```python
from build123d import *

# Parameters (mm, degrees)
BOSS_EXTRUDE1_DEPTH = 3.175
SKETCH3_R           = 1.9685
SKETCH3_R_2         = 1.7018
SKETCH3_R_3         = 1.4605
SKETCH3_R_4         = 1.5875
SKETCH3_R_5         = 1.4732
SKETCH3_R_6         = 1.2065
SKETCH3_W           = 6.5532
SKETCH3_H           = 16.4592
CUT_EXTRUDE1_DEPTH  = 365.434389894


with BuildPart() as part:
    # Sketch1 → Boss-Extrude1 (new body)
    with BuildSketch(Plane(origin=(0, 0, 0), x_dir=(1, 0, 0), z_dir=(0, 1, 0))):
        with BuildLine():
            Line((20.9042, 21.057301381), (20.9042, 9.500301381))
            ThreePointArc((20.9042, 9.500301381), (21.364503799, 7.853774874), (22.611947739, 6.684667206))
            Line((22.611947739, 6.684667206), (32.903843319, 1.321467969))
            add(Edge.make_bspline(
                [(32.903843319, 1.321467969), (33.614873553, 0.950943726), (34.463414094, -1.137550566), (33.907098259, -2.92148302), (32.903843319, -3.444288181)],
                knots=[0, 0, 0, 0, 0.5, 1, 1, 1, 1], degree=3))
            Line((32.903843319, -3.444288181), (22.611947739, -8.807487419))
            ThreePointArc((22.611947739, -8.807487419), (21.364503799, -9.976595087), (20.9042, -11.623121593))
            Line((20.9042, -11.623121593), (20.9042, -27.172610106))
            ThreePointArc((20.9042, -27.172610106), (22.6441, -28.912510106), (24.384, -27.172610106))
            Line((24.384, -27.172610106), (27.051, -27.172610106))
            Line((27.051, -27.172610106), (27.051, -37.859834638))
            ThreePointArc((27.051, -37.859834638), (27.496194931, -39.48118879), (28.706930259, -40.647854028))
            Line((28.706930259, -40.647854028), (80.01, -68.600651316))
            Line((80.01, -68.600651316), (80.01, -252.750651316))
            Line((80.01, -252.750651316), (26.5303, -291.142539353))
            Line((26.5303, -291.142539353), (23.8379, -291.142539353))
            ThreePointArc((23.8379, -291.142539353), (22.1361, -289.440739353), (20.4343, -291.142539353))
            Line((20.4343, -291.142539353), (20.4343, -306.692027866))
            ThreePointArc((20.4343, -306.692027866), (20.894603799, -308.338554372), (22.142047739, -309.50766204))
            Line((22.142047739, -309.50766204), (32.433943319, -314.870861278))
            add(Edge.make_bspline(
                [(32.433943319, -319.63661747), (33.144973553, -319.266093228), (33.993514113, -317.177598915), (33.437198259, -315.393666439), (32.433943319, -314.870861278)],
                knots=[0, 0, 0, 0, 0.5, 1, 1, 1, 1], degree=3))
            Line((32.433943319, -319.63661747), (22.142047738, -324.999816708))
            ThreePointArc((22.142047738, -324.999816708), (20.894603798, -326.168924376), (20.434299999, -327.815450882))
            Line((20.434299999, -327.815450882), (20.434299999, -339.372450882))
            ThreePointArc((20.434299999, -339.372450882), (20.482218455, -339.921983425), (20.62452741, -340.454928408))
            Line((20.62452741, -340.454928408), (23.888699999, -349.455404296))
            Line((23.888699999, -349.455404296), (23.88337128, -351.995398706))
            Line((23.88337128, -351.995398706), (22.237699999, -352.127939395))
            ThreePointArc((22.237699999, -352.127939395), (21.248038856, -351.230539971), (20.451461278, -352.303022636))
            Line((20.451461278, -352.303022636), (20.451461278, -355.528822636))
            Line((20.451461278, -355.528822636), (-20.451461278, -355.528822636))
            Line((-20.451461278, -355.528822636), (-20.451461278, -352.303022636))
            ThreePointArc((-20.451461278, -352.303022636), (-21.248038856, -351.230539971), (-22.237699999, -352.127939395))
            Line((-22.237699999, -352.127939395), (-23.88337128, -351.995398706))
            Line((-23.88337128, -351.995398706), (-23.888699999, -349.455404296))
            Line((-23.888699999, -349.455404296), (-20.62452741, -340.454928408))
            ThreePointArc((-20.62452741, -340.454928408), (-20.482218455, -339.921983425), (-20.434299999, -339.372450882))
            Line((-20.434299999, -339.372450882), (-20.434299999, -327.815450882))
            ThreePointArc((-20.434299999, -327.815450882), (-20.894603798, -326.168924376), (-22.142047738, -324.999816708))
            Line((-22.142047738, -324.999816708), (-32.433943319, -319.63661747))
            add(Edge.make_bspline(
                [(-32.433943319, -319.63661747), (-33.144973553, -319.266093228), (-33.993514113, -317.177598915), (-33.437198259, -315.393666439), (-32.433943319, -314.870861278)],
                knots=[0, 0, 0, 0, 0.5, 1, 1, 1, 1], degree=3))
            Line((-32.433943319, -314.870861278), (-22.142047739, -309.50766204))
            ThreePointArc((-22.142047739, -309.50766204), (-20.894603799, -308.338554372), (-20.4343, -306.692027866))
            Line((-20.4343, -306.692027866), (-20.4343, -291.142539353))
            ThreePointArc((-20.4343, -291.142539353), (-22.1361, -289.440739353), (-23.8379, -291.142539353))
            Line((-23.8379, -291.142539353), (-26.5303, -291.142539353))
            Line((-26.5303, -291.142539353), (-80.01, -252.750651316))
            Line((-80.01, -252.750651316), (-80.01, -68.600651316))
            Line((-80.01, -68.600651316), (-28.706930259, -40.647854028))
            ThreePointArc((-28.706930259, -40.647854028), (-27.496194931, -39.48118879), (-27.051, -37.859834638))
            Line((-27.051, -37.859834638), (-27.051, -27.172610106))
            Line((-27.051, -27.172610106), (-24.384, -27.172610106))
            ThreePointArc((-24.384, -27.172610106), (-22.6441, -28.912510106), (-20.9042, -27.172610106))
            Line((-20.9042, -27.172610106), (-20.9042, -11.623121593))
            ThreePointArc((-20.9042, -11.623121593), (-21.364503799, -9.976595087), (-22.611947739, -8.807487419))
            Line((-22.611947739, -8.807487419), (-32.903843319, -3.444288181))
            add(Edge.make_bspline(
                [(-32.903843319, 1.321467969), (-33.614873553, 0.950943726), (-34.463414094, -1.137550566), (-33.907098259, -2.92148302), (-32.903843319, -3.444288181)],
                knots=[0, 0, 0, 0, 0.5, 1, 1, 1, 1], degree=3))
            Line((-32.903843319, 1.321467969), (-22.611947739, 6.684667206))
            ThreePointArc((-22.611947739, 6.684667206), (-21.364503799, 7.853774874), (-20.9042, 9.500301381))
            Line((-20.9042, 9.500301381), (-20.9042, 21.057301381))
            ThreePointArc((-20.9042, 21.057301381), (-20.952118456, 21.606833923), (-21.094427411, 22.139778906))
            Line((-21.094427411, 22.139778906), (-24.3586, 31.140254794))
            Line((-24.3586, 31.140254794), (-24.3586, 33.680254794))
            Line((-24.3586, 33.680254794), (-22.7076, 33.680254794))
            ThreePointArc((-22.7076, 33.680254794), (-21.8059, 32.778554794), (-20.9042, 33.680254794))
            Line((-20.9042, 33.680254794), (-20.9042, 36.906054794))
            Line((-20.9042, 36.906054794), (20.9042, 36.906054794))
            Line((20.9042, 36.906054794), (20.9042, 33.680254794))
            ThreePointArc((20.9042, 33.680254794), (21.8059, 32.778554794), (22.7076, 33.680254794))
            Line((22.7076, 33.680254794), (24.3586, 33.680254794))
            Line((24.3586, 33.680254794), (24.3586, 31.140254794))
            Line((24.3586, 31.140254794), (21.094427411, 22.139778906))
            ThreePointArc((21.094427411, 22.139778906), (20.952118456, 21.606833923), (20.9042, 21.057301381))
        make_face()
    extrude(amount=BOSS_EXTRUDE1_DEPTH)

    # Sketch3 → Cut-Extrude1 (cut, through all)
    with BuildSketch(Plane(origin=(0, 3.175, 0), x_dir=(1, 0, 0), z_dir=(0, 1, 0))):
        with Locations(Location((-10.0076, 29.870254794, 0), (0, 0, 270))):
            Circle(SKETCH3_R)
        with Locations(Location((10.0076, 29.870254794, 0), (0, 0, 270))):
            Circle(SKETCH3_R)
        with Locations(Location((-10.0076, -10.922145206, 0), (0, 0, 270))):
            Circle(SKETCH3_R)
        with Locations(Location((10.0076, -10.922145206, 0), (0, 0, 270))):
            Circle(SKETCH3_R)
        with Locations(Location((-32.1183, -52.241120441, 0), (0, 0, 270))):
            Circle(SKETCH3_R)
        with Locations(Location((32.1183, -52.241120441, 0), (0, 0, 270))):
            Circle(SKETCH3_R)
        with Locations(Location((-10.0076, -348.493022636, 0), (0, 0, 270))):
            Circle(SKETCH3_R)
        with Locations(Location((10.0076, -348.493022636, 0), (0, 0, 270))):
            Circle(SKETCH3_R)
        with Locations(Location((10.0076, -307.700622636, 0), (0, 0, 270))):
            Circle(SKETCH3_R)
        with Locations(Location((-10.0076, -307.700622636, 0), (0, 0, 270))):
            Circle(SKETCH3_R)
        with Locations(Location((-32.1183, -266.3816474, 0), (0, 0, 270))):
            Circle(SKETCH3_R)
        with Locations(Location((32.1183, -266.3816474, 0), (0, 0, 270))):
            Circle(SKETCH3_R)
        with Locations(Location((-37.409404629, -72.871310848, 0), (0, 0, 270))):
            Circle(SKETCH3_R_2)
        with Locations(Location((-26.982704629, -72.871310848, 0), (0, 0, 270))):
            Circle(SKETCH3_R_3)
        with Locations(Location((-26.982704629, -121.207510848, 0), (0, 0, 270))):
            Circle(SKETCH3_R_3)
        with Locations(Location((-37.409404629, -121.207510848, 0), (0, 0, 270))):
            Circle(SKETCH3_R_2)
        with Locations(Location((37.409404629, -245.751456994, 0), (0, 0, 270))):
            Circle(SKETCH3_R_2)
        with Locations(Location((26.982704629, -245.751456994, 0), (0, 0, 270))):
            Circle(SKETCH3_R_4)
        with Locations(Location((37.409404629, -197.415256994, 0), (0, 0, 270))):
            Circle(SKETCH3_R_2)
        with Locations(Location((26.982704629, -197.415256994, 0), (0, 0, 270))):
            Circle(SKETCH3_R_4)
        with Locations(Location((-10.328284802, -122.607994505, 0), (0, 0, 270))):
            Circle(SKETCH3_R_3)
        with Locations(Location((10.35451602, -196.005997456, 0), (0, 0, 270))):
            Circle(SKETCH3_R_4)
        with Locations(Location((-14.518992261, -139.79255604, 0), (0, 0, 270))):
            Circle(SKETCH3_R)
        with Locations(Location((11.846207739, -139.79255604, 0), (0, 0, 270))):
            Circle(SKETCH3_R)
        with Locations(Location((6.60405639, -177.453267872, 0), (0, 0, 270))):
            Circle(SKETCH3_R)
        with Locations(Location((-19.76114361, -177.453267872, 0), (0, 0, 270))):
            Circle(SKETCH3_R)
        with Locations(Location((75.565, -72.007264101, 0), (0, 0, 270))):
            Circle(SKETCH3_R_3)
        with Locations(Location((-75.565, -72.007264101, 0), (0, 0, 270))):
            Circle(SKETCH3_R_3)
        with Locations(Location((-75.565, -177.036264101, 0), (0, 0, 270))):
            Circle(SKETCH3_R_3)
        with Locations(Location((75.565, -177.036264101, 0), (0, 0, 270))):
            Circle(SKETCH3_R_3)
        with Locations(Location((44.0563, -66.262403585, 0), (0, 0, 270))):
            Circle(SKETCH3_R_5)
        with Locations(Location((55.9943, -194.532403585, 0), (0, 0, 270))):
            Circle(SKETCH3_R_5)
        with Locations(Location((-52.679777995, -130.268623082, 0), (0, 0, 270))):
            Circle(SKETCH3_R_6)
        with Locations(Location((-30.988177995, -130.268623082, 0), (0, 0, 270))):
            Circle(SKETCH3_R_6)
        with Locations(Location((-52.679777995, -160.367623082, 0), (0, 0, 270))):
            Circle(SKETCH3_R_6)
        with Locations(Location((-30.988177995, -160.367623082, 0), (0, 0, 270))):
            Circle(SKETCH3_R_6)
        with Locations((-6.7056, 9.245454794)):
            Rectangle(SKETCH3_W, SKETCH3_H)
        with Locations((6.235699999, -327.868222636)):
            Rectangle(SKETCH3_W, SKETCH3_H)
    extrude(amount=-CUT_EXTRUDE1_DEPTH, mode=Mode.SUBTRACT)


solid = part.part
```
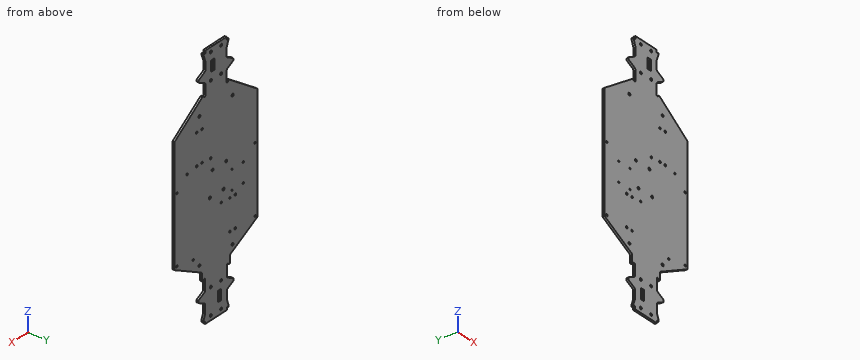
Geometry: final body of the model. Coordinates: model frame, mm. Round coordinates to 2 decimals unless told otherwise and drop trailing zeros. Order: outer loops, then holes, each group sorted by start corner. A loop starts at its lowest first (then second) coordinate and runs counter-clockwise, first axis right, second up. Notation, with made-up numbers: M -1.5,-4 L 9.5,-4 A22 cw 9.5,17 Z; hole C 56,62 d8. An arc over 180 degrees is marked long. Use one line per item in the form item = value. Start each with the question number.
Q1. Material intervals for line 1 (Z direction, x = -11, y = 1.2); line 2 (X direction, y = 2.75, z = -3.5); line 3 (Z direction, x = 28, y = 2.6), sorted ascending. Write a range as [from, to].
Q2. Cut plane B-B (z = 18). Return loops of the section in (x, y) (3 decimals).
Q3. Cut plane A-A (y = 1.1). Count the separate pieces of the cut face and the enclosed holes in it, and give its area (3 significant figures).
Q4. Pin query (flat end, axial travel): pin 1 Ø1 at (x, y) = (47, 2) entering from +Z; pin 2 Ø1 at (y, z) = (2, 331.5) entering from +X; pin 3 Ø1 at (y, z) = (1, -11.5) entering from -X. Return the tip coordinate at first contact, or that it passes through.
Geometry results:
q1.line_1 = [-36.91, -31.57], [-28.17, 9.22], [12.62, 121.31], [123.9, 306], [309.4, 346.79], [350.19, 355.53]
q1.line_2 = [-28.72, -9.98], [-3.43, 28.72]
q1.line_3 = [-3.88, 6], [40.12, 196.2], [198.63, 244.53], [246.97, 290.09], [312.56, 321.95]
q2.outline = M -20.904,0 L 20.904,0 L 20.904,3.175 L -20.904,3.175 Z
q3.separate_pieces = 1
q3.enclosed_holes = 38
q3.area = 42,700 mm^2
q4.pin_1 = 276.81
q4.pin_2 = 20.43
q4.pin_3 = -20.9
